```python
from build123d import *

# Parameters (mm, degrees)
EXTRUDE_5_DEPTH     = 54
SKETCH_10_OUTSIDE_W = 79.172
SKETCH_10_OUTSIDE_H = 73.172
SKETCH_10_OUTSIDE_R = 1.75
CUT_EXTRUDE_1_DEPTH = 4
FILLET_1_R          = 1
EXTRUDE_6_DEPTH     = 65
EXTRUDE_7_DEPTH     = 2


with BuildPart() as part:
    # 草图11 → 凸台-拉伸5 (new body)
    with BuildSketch(Plane.XY):
        with BuildLine():
            Line((-30, 0), (-30, 4))
            Line((-30, 4), (-23.25, 4))
            ThreePointArc((-23.25, 4), (-21.835786438, 4.585786438), (-21.25, 6))
            Line((-21.25, 6), (-21.25, 8))
            ThreePointArc((-21.25, 8), (0, 29.25), (21.25, 8))
            Line((21.25, 8), (21.25, 6))
            ThreePointArc((21.25, 6), (21.835786438, 4.585786438), (23.25, 4))
            Line((23.25, 4), (30, 4))
            Line((30, 4), (30, 0))
            Line((30, 0), (18.25, 0))
            Line((18.25, 0), (18.25, 8))
            ThreePointArc((18.25, 8), (0, 26.25), (-18.25, 8))
            Line((-18.25, 8), (-18.25, 0))
            Line((-18.25, 0), (-30, 0))
        make_face()
    extrude(amount=EXTRUDE_5_DEPTH)

    # 草图10 outside → 切除-拉伸1 (cut)
    with BuildSketch(Plane(origin=(0, 0, 0), x_dir=(1, 0, 0), z_dir=(0, 1, 0))):
        with Locations((0, -27)):
            Rectangle(SKETCH_10_OUTSIDE_W, SKETCH_10_OUTSIDE_H)
        with BuildLine():
            Line((-30, -2), (-30, -52))
            ThreePointArc((-30, -52), (-29.414213562, -53.414213562), (-28, -54))
            Line((-28, -54), (28, -54))
            ThreePointArc((28, -54), (29.414213562, -53.414213562), (30, -52))
            Line((30, -52), (30, -2))
            ThreePointArc((30, -2), (29.414213562, -0.585786438), (28, 0))
            Line((28, 0), (-28, 0))
            ThreePointArc((-28, 0), (-29.414213562, -0.585786438), (-30, -2))
        make_face(mode=Mode.SUBTRACT)
        with Locations((-26, -9)):
            Circle(SKETCH_10_OUTSIDE_R)
        with Locations((26, -9)):
            Circle(SKETCH_10_OUTSIDE_R)
        with Locations((26, -44)):
            Circle(SKETCH_10_OUTSIDE_R)
        with Locations((-26, -44)):
            Circle(SKETCH_10_OUTSIDE_R)
    extrude(amount=CUT_EXTRUDE_1_DEPTH, mode=Mode.SUBTRACT)

    # 圆角1
    fillet_1_edges = [part.edges().sort_by_distance(p)[0] for p in [
        (18.25, 0, 27),
        (-18.25, 0, 27),
    ]]
    fillet(fillet_1_edges, radius=FILLET_1_R)

    # 草图12 → 凸台-拉伸6 (add)
    with BuildSketch(Plane(origin=(0, 0, 0), x_dir=(-1, 0, 0), z_dir=(0, 0, -1))):
        with BuildLine():
            ThreePointArc((-18.25, 8), (0, 26.25), (18.25, 8))
            Line((18.25, 8), (18.25, 6))
            Line((18.25, 6), (18.25, 1))
            ThreePointArc((18.25, 1), (18.542893219, 0.292893219), (19.25, 0))
            Line((19.25, 0), (21.25, 0))
            Line((21.25, 0), (21.25, 6))
            Line((21.25, 6), (21.25, 8))
            ThreePointArc((21.25, 8), (0, 29.25), (-21.25, 8))
            Line((-21.25, 8), (-21.25, 6))
            Line((-21.25, 6), (-21.25, 0))
            Line((-21.25, 0), (-19.25, 0))
            ThreePointArc((-19.25, 0), (-18.542893219, 0.292893219), (-18.25, 1))
            Line((-18.25, 1), (-18.25, 6))
            Line((-18.25, 6), (-18.25, 8))
        make_face()
    extrude(amount=EXTRUDE_6_DEPTH)

    # 草图13 → 凸台-拉伸7 (add)
    with BuildSketch(Plane(origin=(0, 0, -65), x_dir=(-1, 0, 0), z_dir=(0, 0, -1))):
        with BuildLine():
            Line((-18.25, 1), (18.25, 1))
            Line((18.25, 1), (18.25, 8))
            ThreePointArc((18.25, 8), (0, 26.25), (-18.25, 8))
            Line((-18.25, 8), (-18.25, 1))
        make_face()
    extrude(amount=-EXTRUDE_7_DEPTH)


solid = part.part
```
Read the model definition and answer for the solid it produces. Units are mm, in the model's axes. A direction names the side the tool comes from. Round coordinates to 2 decimals unless told otherwise and drop trailing zeros. Write each loop counter-clockwise with the first axis right and the second up, starting at its lowest first coordinate (ties: lowest second). Pieces come first, ordered by that corner, then holes. Notation, with made-up numbers: M 8,3 L 60,3 A28 ccw 60,30 Z; hole C 4,-6 d3. An arc over 180 degrees is marked long. One line per item, written item: value.
Q1. Which of the six approach directions +Z, -Z, +X, -X, +Y, -Y give full straight-line access (tool end or side, diameter ignored) to faces 1 (the flat face through (-21.25, 5, -18)), 2 (the cylindrical face through (0.401, 26.246, -3.681)), 3 (the flat face through (-27, 4, 27))?
Data:
face 1: -Z, -X, +Y
face 2: +Z, -Y
face 3: +Z, -Z, -X, +Y
Q2. Flat-ended cylindrical pins translate along their axes: pin 1 Ø4 at (y, z) = (3, -23) entering from +X; pin 2 Ø3 at (x, z) = (-26, 44) entering from +Y; pin 3 Ø12 at (x, y) = (-2.5, 7.5) entering from +Z; pin 4 Ø12 at (x, z) = (-3, -35.5) entering from -Y. Find the tip coordinate at first contact, or state that the pin passes through.
Data:
pin 1: x = 21.25
pin 2: through
pin 3: z = -63
pin 4: y = 23.88
Q3. Find section C-C on z = -5. Write down the section's boundary in (x, y), plus the area to 3 significant figures.
Data:
outline: M -21.25,0 L -19.25,0 A1 ccw -18.25,1 L -18.25,8 A18.25 cw 18.25,8 L 18.25,1 A1 ccw 19.25,0 L 21.25,0 L 21.25,8 A21.25 ccw -21.25,8 Z
area: 234 mm2
Q4. Find section B-B on z = 9. Write down the section's boundary in (x, y).
Data:
outline: M -30,0 L -27.75,0 L -27.75,4 L -30,4 Z; M -24.25,0 L -19.25,0 A1 ccw -18.25,1 L -18.25,8 A18.25 cw 18.25,8 L 18.25,1 A1 ccw 19.25,0 L 24.25,0 L 24.25,4 L 23.25,4 A2 cw 21.25,6 L 21.25,8 A21.25 ccw -21.25,8 L -21.25,6 A2 cw -23.25,4 L -24.25,4 Z; M 27.75,0 L 30,0 L 30,4 L 27.75,4 Z
Q5. Straight lines are drawn through the part: line 1 (Z direction, x = 26, y = 0.8); line 2 (X direction, y = 1.35, z = 44); line 3 (Z direction, x = 8.5, y = 12.25). For each, find the intervals that lie inside material, in ascending order. Write a range as [from, to].
Data:
line 1: [0, 7.25], [10.75, 42.25], [45.75, 54]
line 2: [-30, -27.75], [-24.25, -18.25], [18.25, 24.25], [27.75, 30]
line 3: [-65, -63]
Q6. Find section D-D on x = 0. Write down the section's boundary in (y, z), plus the area to 4 significant figures.
Data:
outline: M 1,-65 L 29.25,-65 L 29.25,54 L 26.25,54 L 26.25,-63 L 1,-63 Z
area: 407.5 mm2
Q7. Find section A-A on x = -26. Write down the section's boundary in (y, z).
Data:
outline: M 0,0 L 4,0 L 4,7.25 L 0,7.25 Z; M 0,10.75 L 4,10.75 L 4,42.25 L 0,42.25 Z; M 0,45.75 L 4,45.75 L 4,54 L 0,54 Z
Q8. For a pull along Z with two mould halves and no side action, classify faces 4 (the flat face through (25, 2, 0)), 5 (the cylindrical face through (-27.75, 1.97, 8.92)), 6 (the flat face through (-18.25, 5, -4)), 7 (the cylindrical face through (24.25, 1.97, 8.92)) as +Z half, -Z half, draft (parallel to the pull), parting line (faces both ways), or undercut.
Data:
face 4: -Z half
face 5: undercut
face 6: draft
face 7: undercut
